Build history of the part. All positions in model axes, mm. A direction names the side the tool comes from. Round coordinates to 2 decimals unless told otherwise and drop trailing zeros. Loops run counter-clockwise (first coordinate to the right, second up) from the corner with the lowest first, then second, coordinate; pieces in that order, holes last.
from build123d import *

# Parameters (mm, degrees)
F1_DEPTH = 1


with BuildPart() as f1:
    # F0 (on Front) → F1 (new body)
    with BuildSketch(Plane.XZ):
        with BuildLine():
            Line((-55.349811, -4.232354), (-55.349811, -5.232354))
            Line((-55.349811, -5.232354), (0.650189, -5.232354))
            ThreePointArc((0.650189, -5.232354), (0.238892, -4.183401), (-0.770274, -3.682354))
            Line((-0.770274, -3.682354), (-4.912185, -3.297281))
            Line((-4.912185, -3.297281), (-5.349811, -2.85487))
            Line((-5.349811, -2.85487), (-5.861494, -3.209024))
            Line((-5.861494, -3.209024), (-13.912185, -2.460554))
            Line((-13.912185, -2.460554), (-14.349811, -2.018143))
            Line((-14.349811, -2.018143), (-14.861494, -2.372297))
            Line((-14.861494, -2.372297), (-22.912185, -1.623827))
            Line((-22.912185, -1.623827), (-23.349811, -1.181416))
            Line((-23.349811, -1.181416), (-23.861494, -1.53557))
            Line((-23.861494, -1.53557), (-30.349811, -0.932354))
            Line((-30.349811, -0.932354), (-29.349811, -3.432354))
            Line((-29.349811, -3.432354), (-55.349811, -4.232354))
        make_face()
    extrude(amount=F1_DEPTH)


solid = f1.part
(1) Slice it at B-B on x = -16. List the corners of the cut face in (y, z), plus the area to 3 significant figures.
Responses:
outline: (-1, -5.23) - (0, -5.23) - (0, -2.27) - (-1, -2.27) - close
area: 2.97 mm2
(2) Probe line 1 (Z direction, x = -37.5, y = -0.9); line 2 (Z direction, x = -25.5, y = -0.15); line 3 (X direction, y = -0.25, z = -5). List the from-to ranges inside material, lowest first.
Responses:
line 1: z = -5.23 to -3.68
line 2: z = -5.23 to -1.38
line 3: x = -55.35 to 0.63
(3) Slice it at A-A on y = -0.35. List the corners of the cut face in (x, z).
Responses:
outline: (-55.35, -5.23) - (0.65, -5.23) arc R1.57 ccw to (-0.77, -3.68) - (-4.91, -3.3) - (-5.35, -2.85) - (-5.86, -3.21) - (-13.91, -2.46) - (-14.35, -2.02) - (-14.86, -2.37) - (-22.91, -1.62) - (-23.35, -1.18) - (-23.86, -1.54) - (-30.35, -0.93) - (-29.35, -3.43) - (-55.35, -4.23) - close
(4) Pull direction X, two halves, no side cores. Call faces 1 (the face through (0.25, -0.493, -4.195)), 2 (the face through (-22, -1, -4)), 3 (the face through (-27.06, -0.49, -1.24)), 4 (the face through (-55.35, -0.5, -4.7)): +X half, -X half, draft (parallel to the pull), parting line (faces both ways), or undercut.
Responses:
face 1: +X half
face 2: draft
face 3: undercut
face 4: -X half
(5) Which spindle directions (+Z, -Z, +X, -X, +Y, -Y) get a long thin tool onto all of the face, cutting with end or side? Do faces 5 (the face through (-29.86, -0.49, -2.16)), 6 (the face through (-2.812, -0.493, -3.493)), 7 (the face through (-9.83, -0.49, -2.84)). Say none if no direction does.
Responses:
face 5: -X, +Y, -Y
face 6: +Z, +X, +Y, -Y
face 7: +Z, +Y, -Y
(6) Slice it at C-C on x = -27.5. List the corners of the cut face in (y, z).
Responses:
outline: (-1, -5.23) - (0, -5.23) - (0, -1.2) - (-1, -1.2) - close
